Design review of the part shown in the three views and the two pictorial views. Dimensions are in mm from the part's minimum x, y and z. A direction names the side the tool comes from. Coordinates: 2 decimals unless noted, no trailing zeros. Write each loop counter-clockwise with the first axis right and the second up, starting at its lowest first coordinate (ties: lowest second). Pieces come first, ordered by that corner, then holes. Notation, with made-up numbers: M 50.25,57 L 61.25,57 A19 cw 61.25,63 Z; hole C 62,-4.5 d11. An arc over 180 degrees is marked long. Answer as a JSON object with one key per item and string values.
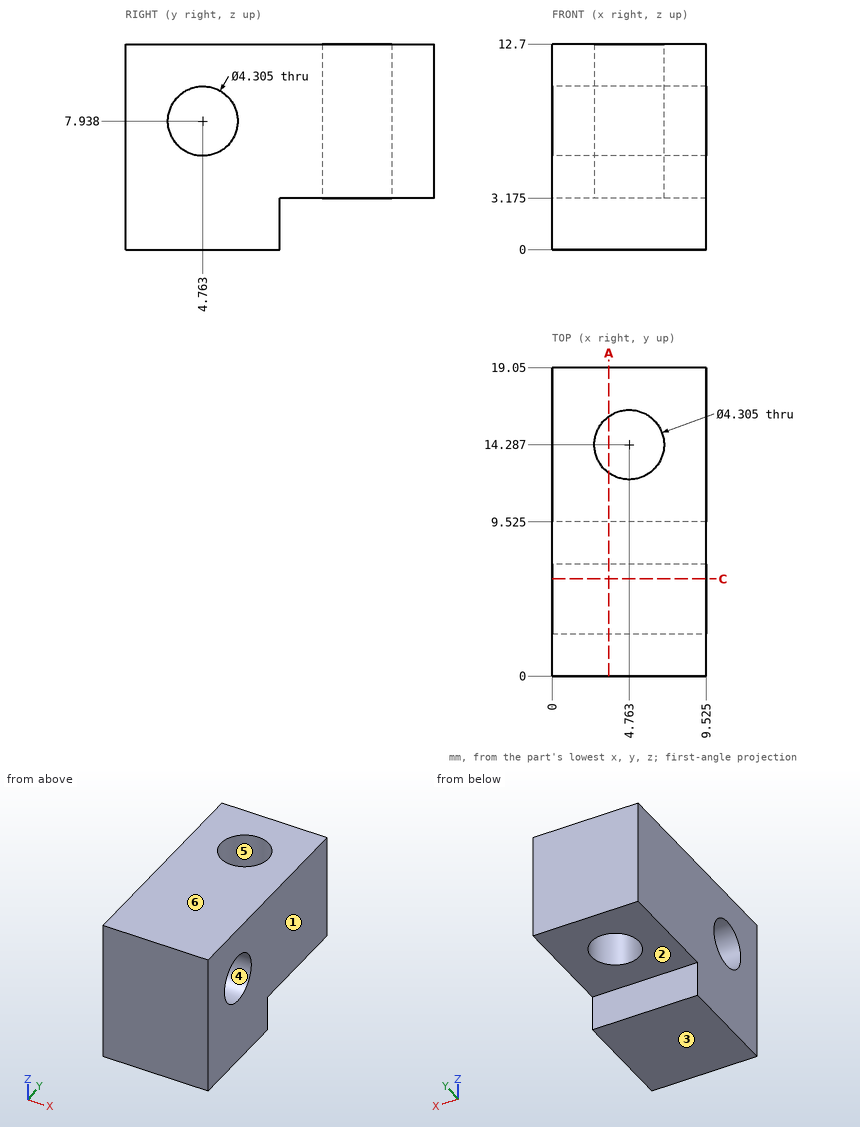
(1) For pin 1 Ø3 at (y, z) = (16, 1.5) entering from +X; pin 2 Ø3 at (x, y) = (7, 14.5) entering from -Z (1 decimal), all flat-tipped, find the tip position at first contact; note any pin that passes through.
Results list:
{"pin 1": "through", "pin 2": "z = 3.2"}
(2) For the marked faces 1 and 2, list the 3-axis set-ups (+Z, -Z, +X, -X, +Y, -Y) from which the entire face can be reached by the end or side of a thin tool; tool diameter is ignored.
Results list:
{"face 1": "+Z, -Z, +X, +Y, -Y", "face 2": "-Z, +X, -X, +Y"}
(3) Wall thickness on line 1 along Y through (x, z) = (3.5, 1.25) (1 decimal); line 2 along Z through (x, y) = (0.5, 3.25) (1 decimal); line 3 along Z through (x, y) = (9, 18) (1 decimal): over which ranges is each line inside the solid? List them lowest first. Write a range as from..to.
Results list:
{"line 1": "0..9.5", "line 2": "0..6.4, 9.5..12.7", "line 3": "3.2..12.7"}
(4) Add section C-C on y = 6. Give the boundary of the cut face in (x, z) (1 decimal).
Results list:
{"outline": "M 0,0 L 9.5,0 L 9.5,6.2 L 0,6.2 Z; M 0,9.7 L 9.5,9.7 L 9.5,12.7 L 0,12.7 Z"}
(5) Draft analysis for pull direction Z (two halves, no side actions). For the marked faces 3, 4, 5 and 6, state which applies: released by +Z, released by -Z, zero draft, split by the parting line, or undercut.
Results list:
{"face 3": "released by -Z", "face 4": "undercut", "face 5": "zero draft", "face 6": "released by +Z"}
(6) Add section A-A on x = 3.5. Count the separate pieces of the cut face and the enclosed holes in it, and give its area (3 significant figures).
Results list:
{"separate pieces": "2", "enclosed holes": "1", "area": "164 mm²"}
